Could you check a few things on this model? Use its own coordinates, in mm. Coordinates: 2 decimals unless noted, no trailing zeros. Order: outer loops, then holes, each group sorted by start corner. A loop starts at its lowest first (then second) coordinate and runs counter-clockwise, first axis right, second up. Notation, with made-up numbers: (49.5, 28.5) -> (94.5, 28.5) arc R29 ccw to (94.5, 53.5) -> close; hole circle Ø1 at (16, 54). An arc over 180 degrees is marked (long way). Put each result on its own line as item: value. Start each with the question number.
Q1. If we section it at A-A (x = 169): Please give me the cut outline in (y, z), and give its area (3 significant figures).
Q2. Will these pins go through, and if not, where does the flat tip stop? pin 1 (18.5 mm diameter, centred on x = 139.47, z = 22.34, fed in from -Y); pin 2 (3.5 mm diameter, centred on x = 148.85, y = 4.19, fed in from -Z).
Q3. Please list where these lines run through material, in increasing order: line 1 along Z through (x, y) = (77, 6.5); line 2 along Z through (x, y) = (162, 3.75); line 3 along X through (y, z) = (5.25, 36.5).
Q4. If we section it at B-B (x = 102): Please give me the cut outline in (y, z), and give its area (3 significant figures).
from build123d import *

# Parameters (mm, degrees)
SKETCH1_W                        = 254
SKETCH1_H                        = 57.15
SKETCH1_R                        = 10
BOSS_EXTRUDE1_DEPTH              = 8
SKETCH25_R                       = 10.25
CUT_EXTRUDE1_DEPTH               = 7.6
SKETCH26_W                       = 254
SKETCH26_H                       = 57.15
BOSS_EXTRUDE2_DEPTH              = 0.4
F_25_0_1495_DIAMETER_HOLE2_D     = 3.7973
F_25_0_1495_DIAMETER_HOLE2_DEPTH = 6.35
F_25_0_1495_DIAMETER_HOLE2_TIP   = 1.140824014
F_25_0_1495_DIAMETER_HOLE1_D     = 3.7973
F_25_0_1495_DIAMETER_HOLE1_DEPTH = 6.35
F_25_0_1495_DIAMETER_HOLE1_TIP   = 1.140824014


with BuildPart() as part:
    # Sketch1 → Boss-Extrude1 (new body)
    with BuildSketch(Plane(origin=(0, 0, 0), x_dir=(1, 0, 0), z_dir=(0, 1, 0))):
        with Locations((92.969183673, -14.086632653)):
            Rectangle(SKETCH1_W, SKETCH1_H)
        with Locations(Location((202.969183673, 0.518367347, 0), (0, 0, 270))):
            Circle(SKETCH1_R, mode=Mode.SUBTRACT)
        with Locations(Location((171.219183673, 0.518367347, 0), (0, 0, 270))):
            Circle(SKETCH1_R, mode=Mode.SUBTRACT)
        with Locations(Location((139.469183673, 0.518367347, 0), (0, 0, 270))):
            Circle(SKETCH1_R, mode=Mode.SUBTRACT)
        with Locations(Location((107.719183673, 0.518367347, 0), (0, 0, 270))):
            Circle(SKETCH1_R, mode=Mode.SUBTRACT)
        with Locations(Location((75.969183673, 0.518367347, 0), (0, 0, 270))):
            Circle(SKETCH1_R, mode=Mode.SUBTRACT)
        with Locations(Location((44.219183673, 0.518367347, 0), (0, 0, 270))):
            Circle(SKETCH1_R, mode=Mode.SUBTRACT)
        with Locations(Location((171.219183673, -22.341632653, 0), (0, 0, 270))):
            Circle(SKETCH1_R, mode=Mode.SUBTRACT)
        with Locations(Location((139.469183673, -22.341632653, 0), (0, 0, 270))):
            Circle(SKETCH1_R, mode=Mode.SUBTRACT)
        with Locations(Location((107.719183673, -22.341632653, 0), (0, 0, 270))):
            Circle(SKETCH1_R, mode=Mode.SUBTRACT)
        with Locations(Location((75.969183673, -22.341632653, 0), (0, 0, 270))):
            Circle(SKETCH1_R, mode=Mode.SUBTRACT)
        with Locations(Location((44.219183673, -22.341632653, 0), (0, 0, 270))):
            Circle(SKETCH1_R, mode=Mode.SUBTRACT)
        with Locations(Location((202.969183673, -22.341632653, 0), (0, 0, 270))):
            Circle(SKETCH1_R, mode=Mode.SUBTRACT)
        with Locations(Location((12.469183673, 0.518367347, 0), (0, 0, 270))):
            Circle(SKETCH1_R, mode=Mode.SUBTRACT)
        with Locations(Location((-19.280816327, 0.518367347, 0), (0, 0, 270))):
            Circle(SKETCH1_R, mode=Mode.SUBTRACT)
        with Locations(Location((12.469183673, -22.341632653, 0), (0, 0, 270))):
            Circle(SKETCH1_R, mode=Mode.SUBTRACT)
        with Locations(Location((-19.280816327, -22.341632653, 0), (0, 0, 270))):
            Circle(SKETCH1_R, mode=Mode.SUBTRACT)
    extrude(amount=BOSS_EXTRUDE1_DEPTH)

    # Sketch25 → Cut-Extrude1 (cut)
    with BuildSketch(Plane.XZ):
        with Locations(Location((44.219183673, 22.341632653, 0), (0, 0, 270))):
            Circle(SKETCH25_R)
        with Locations(Location((75.969183673, 22.341632653, 0), (0, 0, 270))):
            Circle(SKETCH25_R)
        with Locations(Location((107.719183673, 22.341632653, 0), (0, 0, 270))):
            Circle(SKETCH25_R)
        with Locations(Location((139.469183673, 22.341632653, 0), (0, 0, 270))):
            Circle(SKETCH25_R)
        with Locations(Location((171.219183673, 22.341632653, 0), (0, 0, 270))):
            Circle(SKETCH25_R)
        with Locations(Location((202.969183673, 22.341632653, 0), (0, 0, 270))):
            Circle(SKETCH25_R)
        with Locations(Location((75.969183673, -0.518367347, 0), (0, 0, 270))):
            Circle(SKETCH25_R)
        with Locations(Location((107.719183673, -0.518367347, 0), (0, 0, 270))):
            Circle(SKETCH25_R)
        with Locations(Location((139.469183673, -0.518367347, 0), (0, 0, 270))):
            Circle(SKETCH25_R)
        with Locations(Location((171.219183673, -0.518367347, 0), (0, 0, 270))):
            Circle(SKETCH25_R)
        with Locations(Location((202.969183673, -0.518367347, 0), (0, 0, 270))):
            Circle(SKETCH25_R)
        with Locations(Location((44.219183673, -0.518367347, 0), (0, 0, 270))):
            Circle(SKETCH25_R)
        with Locations(Location((12.469183673, 22.341632653, 0), (0, 0, 270))):
            Circle(SKETCH25_R)
        with Locations(Location((-19.280816327, 22.341632653, 0), (0, 0, 270))):
            Circle(SKETCH25_R)
        with Locations(Location((-19.280816327, -0.518367347, 0), (0, 0, 270))):
            Circle(SKETCH25_R)
        with Locations(Location((12.469183673, -0.518367347, 0), (0, 0, 270))):
            Circle(SKETCH25_R)
    extrude(amount=-CUT_EXTRUDE1_DEPTH, mode=Mode.SUBTRACT)

    # Sketch26 → Boss-Extrude2 (add)
    with BuildSketch(Plane(origin=(0, 8, 0), x_dir=(1, 0, 0), z_dir=(0, 1, 0))):
        with Locations((92.969183673, -14.086632653)):
            Rectangle(SKETCH26_W, SKETCH26_H)
    extrude(amount=-BOSS_EXTRUDE2_DEPTH)

    # #25 (0.1495) Diameter Hole2
    with Locations(Plane.XY.offset(42.661632653)):
        with Locations((15.499183673, 5.968), (162.819183673, 5.968), (89.159183673, 5.968)):
            Hole(F_25_0_1495_DIAMETER_HOLE2_D / 2, depth=F_25_0_1495_DIAMETER_HOLE2_DEPTH)
            with Locations((0, 0, -(F_25_0_1495_DIAMETER_HOLE2_DEPTH + F_25_0_1495_DIAMETER_HOLE2_TIP / 2))):  # 118° drill point
                Cone(0, F_25_0_1495_DIAMETER_HOLE2_D / 2, F_25_0_1495_DIAMETER_HOLE2_TIP, mode=Mode.SUBTRACT)

    # #25 (0.1495) Diameter Hole1
    with Locations(Plane(origin=(0, 0, -14.488367347), x_dir=(-1, 0, 0), z_dir=(0, 0, -1))):
        with Locations((-148.849183673, 4.19), (-85.349183673, 4.19), (-21.849183673, 4.19)):
            Hole(F_25_0_1495_DIAMETER_HOLE1_D / 2, depth=F_25_0_1495_DIAMETER_HOLE1_DEPTH)
            with Locations((0, 0, -(F_25_0_1495_DIAMETER_HOLE1_DEPTH + F_25_0_1495_DIAMETER_HOLE1_TIP / 2))):  # 118° drill point
                Cone(0, F_25_0_1495_DIAMETER_HOLE1_D / 2, F_25_0_1495_DIAMETER_HOLE1_TIP, mode=Mode.SUBTRACT)


solid = part.part
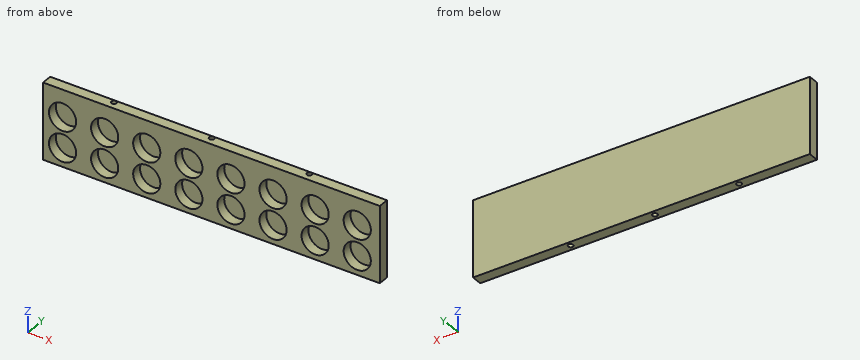
The answers:
1. outline: (0, -14.49) -> (8, -14.49) -> (8, 42.66) -> (0, 42.66) -> (0, 32.35) -> (7.6, 32.35) -> (7.6, 12.33) -> (0, 12.33) -> (0, 9.49) -> (7.6, 9.49) -> (7.6, -10.53) -> (0, -10.53) -> close
1. area: 153 mm^2
2. pin 1: y = 7.6
2. pin 2: z = -8.05
3. line 1: -14.49 to -10.72, 9.68 to 12.14, 32.54 to 42.66
3. line 2: -14.49 to -5, 3.96 to 17.86, 26.82 to 42.66
3. line 3: -34.03 to 13.74, 17.26 to 87.4, 90.92 to 161.06, 164.58 to 219.97
4. outline: (0, -14.49) -> (8, -14.49) -> (8, 42.66) -> (0, 42.66) -> (0, 30.85) -> (7.6, 30.85) -> (7.6, 13.84) -> (0, 13.84) -> (0, 7.99) -> (7.6, 7.99) -> (7.6, -9.02) -> (0, -9.02) -> close
4. area: 199 mm^2
